Geometry check sheet. Reference: drawing and pictorial views, mm from the part's lowest x, y, z. A direction names the side the tool comes from. Give positions to 0.01 mm unless a question says otherwise; leave off trailing zeros. Write each loop counter-clockwise with the first axis right and the second up, starting at its lowest first coordinate (ties: lowest second). Pieces come first, ordered by that corner, then holes. Notation, with made-up numbers: (24.25, 45.5) - (35.25, 45.5) arc R20 ccw to (35.25, 57.5) - close; hole circle Ø2 at (17, -37). An arc over 180 degrees is marked (long way). Write item = value, one per line. Start each with the question number.
(1) Section check A-A, the plane z = 4. Enter the section's corners in (x, y), plus the area to 3 significant figures.
(2) Access from +Z, -Z, +X, -X, +Y, -Y to the whole of each face (thin tool, end or side, straight path). Record for the marked faces 5, 6 and 7.
(3) Draft check along X on the marked faces 1, 2, 3 and 4. Enter one of: pulls with the +X half, pulls with the -X half, needs draft (parallel to the pull), parting line crosses it, or undercut.
(4) Section check C-C, the plane y = 7. Enter the section's corners in (x, z).
(5) Depth check by flat-ended pin: pin 1 Ø1.5 at (y, z) = (6.5, 3.5) entering from -X; pin 2 Ø2.5 at (x, z) = (17, 2) entering from -Y; pin 3 Ø3 at (y, z) = (3.5, 4.5) entering from +X; pin 4 Ø3 at (y, z) = (3, 5) entering from -X. Enter the tip coordinate at first touch or a pass-through.
(6) Section check B-B, the plane x = 9.95. Enter the section's corners in (y, z), plus the area to 3 significant figures.
(7) Thickness scan on L1, parallel to X at y = 5.75, z = 4; L2, parallel to Z at x = 9.95, y = 11.25; L3, parallel to X at y = 9, z = 4. Record the ranges inside material, lowest first.
(8) Section check D-D, the plane z = 7.5. Enter the section's corners in (x, y).
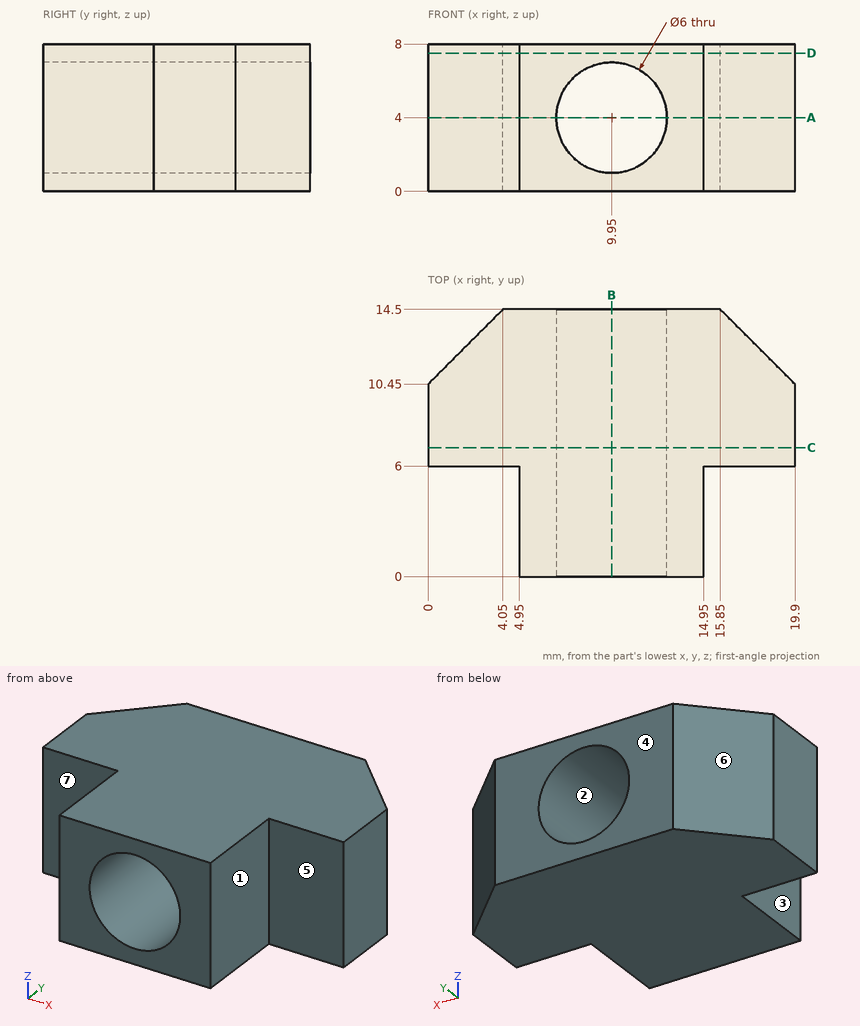
Model answer:
q1.outline = (0, 6) - (4.95, 6) - (4.95, 0) - (6.95, 0) - (6.95, 14.5) - (4.05, 14.5) - (0, 10.45) - close; (12.95, 0) - (14.95, 0) - (14.95, 6) - (19.9, 6) - (19.9, 10.45) - (15.85, 14.5) - (12.95, 14.5) - close
q1.area = 126 mm²
q2.face_5 = +Z, -Z, +X, -Y
q2.face_6 = +Z, -Z, -X, +Y
q2.face_7 = +Z, -Z, -X, -Y
q3.face_1 = pulls with the +X half
q3.face_2 = undercut
q3.face_3 = pulls with the -X half
q3.face_4 = needs draft
q4.outline = (0, 0) - (19.9, 0) - (19.9, 8) - (0, 8) - close; hole circle Ø6 at (9.95, 4)
q5.pin_1 = 0
q5.pin_2 = 6
q5.pin_3 = 14.95
q5.pin_4 = 4.95
q6.outline = (0, 0) - (14.5, 0) - (14.5, 1) - (0, 1) - close; (0, 7) - (14.5, 7) - (14.5, 8) - (0, 8) - close
q6.area = 29.0 mm²
q7.L1 = 4.95 to 6.95, 12.95 to 14.95
q7.L2 = 0 to 1, 7 to 8
q7.L3 = 0 to 6.95, 12.95 to 19.9
q8.outline = (0, 6) - (4.95, 6) - (4.95, 0) - (14.95, 0) - (14.95, 6) - (19.9, 6) - (19.9, 10.45) - (15.85, 14.5) - (4.05, 14.5) - (0, 10.45) - close
